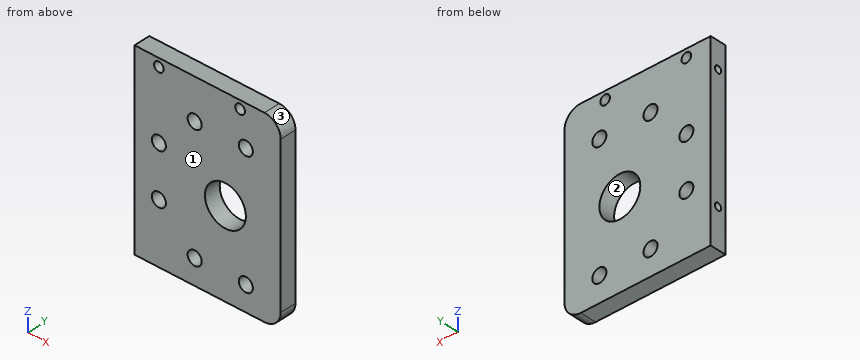
```python
from build123d import *

# Parameters (mm, degrees)
SKETCH1_W                     = 57.15
SKETCH1_H                     = 73.66
BOSS_EXTRUDE1_DEPTH           = 6.35
F_6_CLEARANCE_HOLE1_D         = 3.7973
F_6_CLEARANCE_HOLE1_DEPTH     = 12.7
F_6_CLEARANCE_HOLE1_TIP       = 1.140824014
M5_CLEARANCE_HOLE1_D          = 5.5
M5_CLEARANCE_HOLE1_DEPTH      = 12.7
M5_CLEARANCE_HOLE1_TIP        = 1.652366702
SKETCH6_R                     = 8
CUT_EXTRUDE1_DEPTH            = 6.35
TAP_DRILL_FOR_6_32_TAP1_D     = 2.7051
TAP_DRILL_FOR_6_32_TAP1_DEPTH = 12.7
TAP_DRILL_FOR_6_32_TAP1_TIP   = 0.81269403
FILLET1_R                     = 6.35


with BuildPart() as part:
    # Sketch1 → Boss-Extrude1 (new body)
    with BuildSketch(Plane(origin=(0, 0, 0), x_dir=(1, 0, 0), z_dir=(0, 1, 0))):
        Rectangle(SKETCH1_W, SKETCH1_H)
    extrude(amount=BOSS_EXTRUDE1_DEPTH)

    # #6 Clearance Hole1
    with Locations(Plane(origin=(0, 6.35, 0), x_dir=(1, 0, 0), z_dir=(0, 1, 0))):
        with Locations((-19.05, -33.655), (12.7, -33.655)):
            Hole(F_6_CLEARANCE_HOLE1_D / 2, depth=F_6_CLEARANCE_HOLE1_DEPTH)
            with Locations((0, 0, -(F_6_CLEARANCE_HOLE1_DEPTH + F_6_CLEARANCE_HOLE1_TIP / 2))):  # 118° drill point
                Cone(0, F_6_CLEARANCE_HOLE1_D / 2, F_6_CLEARANCE_HOLE1_TIP, mode=Mode.SUBTRACT)

    # M5 Clearance Hole1
    with Locations(Plane(origin=(0, 6.35, 0), x_dir=(1, 0, 0), z_dir=(0, 1, 0))):
        with Locations((-19.05, 13.045000006), (-19.05, -6.954999994), (6.95, 3.045000006), (14.95, 27.045), (14.95, -20.955), (-5.05, 27.045), (-5.05, -20.955)):
            Hole(M5_CLEARANCE_HOLE1_D / 2, depth=M5_CLEARANCE_HOLE1_DEPTH)
            with Locations((0, 0, -(M5_CLEARANCE_HOLE1_DEPTH + M5_CLEARANCE_HOLE1_TIP / 2))):  # 118° drill point
                Cone(0, M5_CLEARANCE_HOLE1_D / 2, M5_CLEARANCE_HOLE1_TIP, mode=Mode.SUBTRACT)

    # Sketch6 → Cut-Extrude1 (cut)
    with BuildSketch(Plane(origin=(0, 6.35, 0), x_dir=(1, 0, 0), z_dir=(0, 1, 0))):
        with Locations(Location((6.95, 3.045000006, 0), (0, 0, 270))):
            Circle(SKETCH6_R)
    extrude(amount=-CUT_EXTRUDE1_DEPTH, mode=Mode.SUBTRACT)

    # Tap Drill for #6-32 Tap1
    with Locations(Plane.ZY.offset(28.575)):
        with Locations((26.67, 3.175), (-21.59, 3.175)):
            Hole(TAP_DRILL_FOR_6_32_TAP1_D / 2, depth=TAP_DRILL_FOR_6_32_TAP1_DEPTH)
            with Locations((0, 0, -(TAP_DRILL_FOR_6_32_TAP1_DEPTH + TAP_DRILL_FOR_6_32_TAP1_TIP / 2))):  # 118° drill point
                Cone(0, TAP_DRILL_FOR_6_32_TAP1_D / 2, TAP_DRILL_FOR_6_32_TAP1_TIP, mode=Mode.SUBTRACT)

    # Fillet1
    fillet1_edges = [part.edges().sort_by_distance(p)[0] for p in [
        (28.575, 3.175, -36.83),
        (28.575, 3.175, 36.83),
    ]]
    fillet(fillet1_edges, radius=FILLET1_R)


solid = part.part
```
Verification items for the finished model (mm, model axes). Face numbers are marked on the shaded views. Coordinates: 2 decimals unless noted, no trailing zeros. Loops run counter-clockwise (first coordinate to the right, second up) from the corner with the lowest first, then second, coordinate; pieces in that order, holes last. Notation, with made-up numbers: (46, 71) -> (55, 71) arc R22 cw to (55, 82) -> close; hole circle Ø6 at (77, 22). An arc over 180 degrees is marked (long way). Answer in a Markdown table with one row per item. Add a question column.
1. Section check C-C, the plane z = -15. Enter the section's corners in (x, y) (3 decimals), then the cut area to 3 significant figures.
2. Draft check along X on the marked faces 1, 2 and 3. Enter one of: +X half, -X half, draft (parallel to the pull), parting line (faces both ways), or undercut.
3. Section check D-D, the plane x = -5.05. Enter the section's corners in (y, z) (3 decimals).
4. Depth check by flat-ended pin: P1, Ø1.6, axis at y = 3.175, z = 26.67, coming from the -X side; P2, Ø4.5, axis at x = -19.05, z = 33.655, coming from the -Y side. Enter the tip coordinate at first touch or a pass-through.
5. Section check A-A, the plane x = 6.95. Enter the section's corners in (y, z) (3 decimals).
6. Section check B-B, the plane x = -19.05. Enter the section's corners in (y, z) (3 decimals).
7. Material ranges on probe 1 along X at (y, z) = (5.5, -27) (3 decimals); probe 2 along X at (y, z) = (2, -13) (3 decimals); probe 3 along Z at (x, y) = (6.5, 3), recorded low to high. Write a range as [from, to].
Derived:
| question | item | result |
|---|---|---|
| 1 | outline | (-28.575, 0) -> (-20.984, 0) -> (-20.984, 6.35) -> (-28.575, 6.35) -> close; (-17.116, 0) -> (28.575, 0) -> (28.575, 6.35) -> (-17.116, 6.35) -> close |
| 1 | area | 338 mm² |
| 2 | face 1 | draft |
| 2 | face 2 | undercut |
| 2 | face 3 | +X half |
| 3 | outline | (0, -36.83) -> (6.35, -36.83) -> (6.35, -29.795) -> (0, -29.795) -> close; (0, -24.295) -> (6.35, -24.295) -> (6.35, 18.205) -> (0, 18.205) -> close; (0, 23.705) -> (6.35, 23.705) -> (6.35, 36.83) -> (0, 36.83) -> close |
| 4 | P1 | stops at x = -15.54 |
| 4 | P2 | stops at y = 0 |
| 5 | outline | (0, -36.83) -> (6.35, -36.83) -> (6.35, -11.045) -> (0, -11.045) -> close; (0, 4.955) -> (6.35, 4.955) -> (6.35, 36.83) -> (0, 36.83) -> close |
| 6 | outline | (0, -36.83) -> (6.35, -36.83) -> (6.35, -15.795) -> (0, -15.795) -> close; (0, -10.295) -> (6.35, -10.295) -> (6.35, 4.205) -> (0, 4.205) -> close; (0, 9.705) -> (6.35, 9.705) -> (6.35, 31.756) -> (0, 31.756) -> close; (0, 35.554) -> (6.35, 35.554) -> (6.35, 36.83) -> (0, 36.83) -> close; hole circle Ø2.705 at (3.175, -21.59); hole circle Ø2.705 at (3.175, 26.67) |
| 7 | probe 1 | x = [-28.575, -7.8], [-2.3, 12.2], [17.7, 28.575] |
| 7 | probe 2 | x = [-28.575, -21.8], [-16.3, 28.575] |
| 7 | probe 3 | z = [-36.83, -11.03], [4.94, 36.83] |
